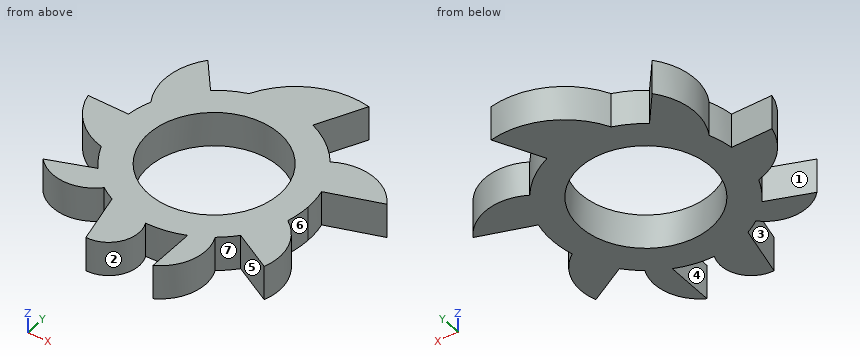
from build123d import *

# Parameters (mm, degrees)
F0_R     = 13.2
F1_DEPTH = 7


with BuildPart() as f1:
    # F0 (on Top) → F1 (new body)
    with BuildSketch(Plane.XY):
        with BuildLine():
            ThreePointArc((18.310132, -4.740264), (18.76226, -2.389272), (18.913779, 0))
            ThreePointArc((18.913779, 0), (18.775293, 2.284599), (18.361864, 4.535742))
            ThreePointArc((18.361864, 4.535742), (17.037777, 8.212501), (14.986336, 11.538663))
            ThreePointArc((14.986336, 11.538663), (11.456299, 15.049393), (7.13248, 17.517384))
            ThreePointArc((7.13248, 17.517384), (0.571768, 18.905134), (-6.060819, 17.916403))
            ThreePointArc((-6.060819, 17.916403), (-8.967974, 16.652521), (-11.623212, 14.920857))
            ThreePointArc((-11.623212, 14.920857), (-15.214001, 11.236778), (-17.679205, 6.721363))
            ThreePointArc((-17.679205, 6.721363), (-18.38519, 4.440249), (-18.798132, 2.088361))
            ThreePointArc((-18.798132, 2.088361), (-18.725211, -2.664116), (-17.469759, -7.248349))
            ThreePointArc((-17.469759, -7.248349), (-16.186317, -9.784385), (-14.537336, -12.099458))
            ThreePointArc((-14.537336, -12.099458), (-12.794361, -13.929657), (-10.822932, -15.51113))
            ThreePointArc((-10.822932, -15.51113), (-9.4883, -16.361638), (-8.087237, -17.097591))
            ThreePointArc((-8.087237, -17.097591), (-4.144332, -18.454147), (0, -18.913779))
            ThreePointArc((0, -18.913779), (3.76722, -18.534807), (7.383474, -17.41308))
            ThreePointArc((7.383474, -17.41308), (9.410528, -16.406492), (11.302837, -15.164989))
            ThreePointArc((11.302837, -15.164989), (12.902521, -13.829533), (14.345584, -12.326202))
            ThreePointArc((14.345584, -12.326202), (16.762624, -8.760449), (18.310132, -4.740264))
        make_face()
        Circle(F0_R, mode=Mode.SUBTRACT)
        with BuildLine():
            ThreePointArc((14.986336, 11.538663), (17.037777, 8.212501), (18.361864, 4.535742))
            Line((18.361864, 4.535742), (28.862666, 8.188942))
            ThreePointArc((28.862666, 8.188942), (22.606509, 12.689041), (14.986336, 11.538663))
        make_face()
        with BuildLine():
            ThreePointArc((22.15042, -16.512131), (22.234177, -9.972473), (18.310132, -4.740264))
            ThreePointArc((18.310132, -4.740264), (16.762624, -8.760449), (14.345584, -12.326202))
            Line((14.345584, -12.326202), (22.15042, -16.512131))
        make_face()
        with BuildLine():
            ThreePointArc((-6.060819, 17.916403), (0.571768, 18.905134), (7.13248, 17.517384))
            Line((7.13248, 17.517384), (11.679311, 26.714748))
            ThreePointArc((11.679311, 26.714748), (1.325059, 25.308147), (-6.060819, 17.916403))
        make_face()
        with BuildLine():
            ThreePointArc((7.383474, -26.983239), (11.671181, -21.846172), (11.302837, -15.164989))
            ThreePointArc((11.302837, -15.164989), (9.410528, -16.406492), (7.383474, -17.41308))
            Line((7.383474, -17.41308), (7.383474, -26.983239))
        make_face()
        with BuildLine():
            ThreePointArc((-17.679205, 6.721363), (-15.214001, 11.236778), (-11.623212, 14.920857))
            Line((-11.623212, 14.920857), (-16.517041, 20.883616))
            ThreePointArc((-16.517041, 20.883616), (-19.358616, 13.987987), (-17.679205, 6.721363))
        make_face()
        with BuildLine():
            ThreePointArc((-5.681629, -27.615353), (-0.414558, -24.848773), (0, -18.913779))
            ThreePointArc((0, -18.913779), (-4.144332, -18.454147), (-8.087237, -17.097591))
            Line((-8.087237, -17.097591), (-5.681629, -27.615353))
        make_face()
        with BuildLine():
            ThreePointArc((-17.469759, -7.248349), (-18.725211, -2.664116), (-18.798132, 2.088361))
            Line((-18.798132, 2.088361), (-26.958849, 2.088361))
            ThreePointArc((-26.958849, 2.088361), (-23.510173, -3.897012), (-17.469759, -7.248349))
        make_face()
        with BuildLine():
            ThreePointArc((-23.224378, -15.438171), (-17.039334, -18.139689), (-10.822932, -15.51113))
            ThreePointArc((-10.822932, -15.51113), (-12.794361, -13.929657), (-14.537336, -12.099458))
            Line((-14.537336, -12.099458), (-23.224378, -15.438171))
        make_face()
    extrude(amount=F1_DEPTH)


solid = f1.part
Could you check a few things on this model? Use its own coordinates, in mm. Face numbers are marked on the shaded views. A direction names the side the tool comes from. Coordinates: 2 decimals unless noted, no trailing zeros. Loops run counter-clockwise (first coordinate to the right, second up) from the corner with the lowest first, then second, coordinate; pieces in that order, holes last.
1. Imagine slicing it at D-D (x = -3.5). Please give me the cut outline in (y, z).
2. Imagine slicing it at A-A (x = 9.5). Please give me the cut outline in (y, z).
3. Imagine slicing it at B-B (z = 1.5). Please give me the cut outline in (x, y), and give its area (3 significant figures).
4. We'd pull the mould along Y, two halves only. Please class the marked faces 1, 2, 3 and 4: released by +Y, released by -Y, zero draft, split by the parting line, or undercut.
5. Imagine slicing it at C-C (y = -6). Please give me the cut outline in (x, z).
6. For the marked faces 5, 6 and 7, which set-ups out of +Z, -Z, +X, -X, +Y, -Y let a thin tool reach every point of the face, with its end or its side?
7. I need wall thicknesses on L1, parallel to X at y = 11.5, z = 3; L2, parallel to X at y = -21, z = 3.25; L3, parallel to Y at x = -16, z = 5.5. Which ranges of each line are inside material? Lowest first, please.
8. For P1, Ø3, axis at x = -2.5, z = 2.5, coming from the -Y side; P2, Ø1, axis at x = -16.5, z = 5, coming from the -Y side; P3, Ø3.5, axis at x = -22.5, z = 2.5, coming from the +Y side; P4, Ø21, axis at x = 0, y = 0, coming from the -Z side, each with a flat end and sliding along its axis, tell me the tip position at first contact or that it passes through.
Computed values:
1. outline: (-27.27, 0) - (-12.73, 0) - (-12.73, 7) - (-27.27, 7) - close; (12.73, 0) - (21.67, 0) - (21.67, 7) - (12.73, 7) - close
2. outline: (-25.39, 0) - (-9.16, 0) - (-9.16, 7) - (-25.39, 7) - close; (9.16, 0) - (16.35, 0) - (16.35, 7) - (9.16, 7) - close; (22.31, 0) - (26.98, 0) - (26.98, 7) - (22.31, 7) - close
3. outline: (-26.96, 2.09) arc R12.91 ccw to (-17.47, -7.25) arc R18.91 ccw to (-14.54, -12.1) - (-23.22, -15.44) arc R8.55 ccw to (-10.82, -15.51) arc R18.91 ccw to (-8.09, -17.1) - (-5.68, -27.62) arc R6.11 ccw to (0, -18.91) arc R18.91 ccw to (7.38, -17.41) - (7.38, -26.98) arc R9.13 ccw to (11.3, -15.16) arc R18.91 ccw to (14.35, -12.33) - (22.15, -16.51) arc R10.15 ccw to (18.31, -4.74) arc R18.91 ccw to (18.91, 0) arc R18.91 ccw to (18.36, 4.54) - (28.86, 8.19) arc R10.22 ccw to (14.99, 11.54) arc R18.91 ccw to (7.13, 17.52) - (11.68, 26.71) arc R16.34 ccw to (-6.06, 17.92) arc R18.91 ccw to (-11.62, 14.92) - (-16.52, 20.88) arc R12.26 ccw to (-17.68, 6.72) arc R18.91 ccw to (-18.8, 2.09) - close; hole circle Ø26.4 at (0, 0)
3. area: 1,040 mm2
4. face 1: undercut
4. face 2: undercut
4. face 3: released by -Y
4. face 4: zero draft
5. outline: (-20.69, 0) - (-11.76, 0) - (-11.76, 7) - (-20.69, 7) - close; (11.76, 0) - (19.82, 0) - (19.82, 7) - (11.76, 7) - close
6. face 5: +Z, -Z, -Y
6. face 6: +Z, -Z, +X
6. face 7: +Z, -Z
7. L1: x = -19.31 to -6.48, 6.48 to 25.5
7. L2: x = -7.19 to 0.56, 7.38 to 11.91
7. L3: y = -18.08 to -12.66, -10.09 to 20.25
8. P1: stops at y = -27.42
8. P2: stops at y = -18.14
8. P3: stops at y = 2.09
8. P4: passes through
